```python
from build123d import *

# Parameters (mm, degrees)
F2_DEPTH = 38.1
F1_R     = 4.191664
F1_R_2   = 4.888278
F3_DEPTH = 38.1


with BuildPart() as f2:
    # F0 (on Front) → F2 (new body, symmetric)
    with BuildSketch(Plane.XZ):
        with BuildLine():
            Line((-53.521972, 29.483171), (-62.049322, 22.979138))
            Line((-62.049322, 22.979138), (-62.049322, -17.520668))
            Line((-62.049322, -17.520668), (-53.521972, -23.408599))
            Line((-53.521972, -23.408599), (-26.112633, -23.408599))
            Line((-26.112633, -23.408599), (-16.773155, -14.272154))
            Line((-16.773155, -14.272154), (1.499737, -21.175247))
            ThreePointArc((1.499737, -21.175247), (19.255094, -20.912232), (17.705545, -3.222666))
            Line((17.705545, -3.222666), (32.90997, 25.973593))
            ThreePointArc((32.90997, 25.973593), (50.002283, 33.973494), (41.596282, 50.869786))
            Line((41.596282, 50.869786), (15.718478, 59.210562))
            Line((15.718478, 59.210562), (-27.696349, 29.483171))
            Line((-27.696349, 29.483171), (-53.521972, 29.483171))
        make_face()
    extrude(amount=F2_DEPTH, both=True)

    # F1 (on face) → F3 (cut, symmetric)
    with BuildSketch(Plane.XZ):
        with Locations((10.020046, -12.490342)):
            Circle(F1_R)
        with Locations((38.078971, 39.35767)):
            Circle(F1_R_2)
        Polygon((-46.49493, -13.530695), (-34.363216, -6.82854), (-34.101594, 7.02891), (-45.971688, 14.184206), (-58.103403, 7.482052), (-58.365024, -6.375399), align=None)
    extrude(amount=F3_DEPTH, both=True, mode=Mode.SUBTRACT)


solid = f2.part
```
Here's how the part is built. I have some questions about the finished solid (model axes, mm). A direction names the side the tool comes from. Round coordinates to 2 decimals unless told otherwise and drop trailing zeros. Order: outer loops, then holes, each group sorted by start corner. A loop starts at its lowest first (then second) coordinate and runs counter-clockwise, first axis right, second up. Notation, with made-up numbers: M -8.75,79.5 L 49.25,79.5 A31 cw 49.25,104.5 Z; hole C 4.25,33.5 d4. An arc over 180 degrees is marked long. Use CSV: the item, a comma, the result in double quotes.
1) If we mould it in two halves opening along Z, with no side actions, what happens to faces 1 (the cylindrical face through (19.066, -0.533, -21.117)), 2 (the flat face through (-5.69, -0.53, 44.55)), 3 (the flat face through (-21.508, -0.533, -18.904)), 4 (the flat face through (25.2, -0.53, 11.17))? For each: pulls with the +Z half, pulls with the -Z half, needs draft (parallel to the pull), parting line crosses it, or undercut.
Taken from the geometry:
face 1,"undercut"
face 2,"pulls with the +Z half"
face 3,"pulls with the -Z half"
face 4,"undercut"
2) I want a section at B-B (x = 39.5). List the corners of the cut face in (y, z) for me.
Taken from the geometry:
outline,"M -38.1,25.27 L 38.1,25.27 L 38.1,34.68 L -38.1,34.68 Z; M -38.1,44.03 L 38.1,44.03 L 38.1,51.55 L -38.1,51.55 Z"
3) I want a section at C-C (y = 25). List the corners of the cut face in (x, z) for me, then the cut area to 3 significant figures.
Taken from the geometry:
outline,"M -62.05,-17.52 L -53.52,-23.41 L -26.11,-23.41 L -16.77,-14.27 L 1.5,-21.18 A12.12 ccw long 17.71,-3.22 L 32.91,25.97 A13.19 ccw long 41.6,50.87 L 15.72,59.21 L -27.7,29.48 L -53.52,29.48 L -62.05,22.98 Z; hole M -58.37,-6.38 L -46.49,-13.53 L -34.36,-6.83 L -34.1,7.03 L -45.97,14.18 L -58.1,7.48 Z; hole C 10.02,-12.49 d8.38; hole C 38.08,39.36 d9.78"
area,"5,250 mm^2"
4) I want a section at A-A (z = 37.5). List the corners of the cut face in (x, y) for me.
Taken from the geometry:
outline,"M -15.99,-38.1 L 33.56,-38.1 L 33.56,38.1 L -15.99,38.1 Z; M 42.6,-38.1 L 50.71,-38.1 L 50.71,38.1 L 42.6,38.1 Z"
5) On a 3-axis mill with a long thin cutter (end or side, diameter ignored), from which of +Z, -Z, +X, -X, +Y, -Y can I reach the whole of each face in a straight line? I mean faces 5 (the flat face through (-6, -38.1, 18)), 6 (the flat face through (-6, 38.1, 18)), 7 (the flat face through (-40, -1, -23.409)), 8 (the flat face through (-51.95, -0.53, 10.88)), 9 (the flat face through (-7.765, -0.533, -17.675)). Say none if no direction works.
Taken from the geometry:
face 5,"+Z, -Z, +X, -X, -Y"
face 6,"+Z, -Z, +X, -X, +Y"
face 7,"-Z, -X, +Y, -Y"
face 8,"+Y, -Y"
face 9,"-Z, +Y, -Y"
6) I'm going to push flat-ended pins straight in: P1, Ø5, axis at y = -14, z = 33.5, coming from the -X side; P2, Ø8, axis at x = -39, y = -18.5, coming from the -Z side; P3, Ø5, axis at x = 32, y = -21, coming from the +Z side; P4, Ø12.5, axis at x = 38.08, z = 39.36, coming from the -Y side. Where does each tip first touch, or does it pass through?
Taken from the geometry:
P1,"x = -25.48"
P2,"z = -23.41"
P3,"z = 54.77"
P4,"y = -38.1"
7) I need wall thicknesses on line 1 along X through (y, z) = (-29.5, -12); line 2 along X through (y, z) = (7.5, -10.5); line 3 along Z through (x, y) = (36, -15.5). Which ranges of each line are inside material? Lowest first, please. Write a range as [from, to].
Taken from the geometry:
line 1,"[-62.05, -49.03], [-43.72, 5.86], [14.18, 22.35]"
line 2,"[-62.05, -51.52], [-41.01, 6.33], [13.71, 22.16]"
line 3,"[25.22, 34.93], [43.78, 52.67]"
8) I want a section at D-D (z = 18.5). List the corners of the cut face in (x, y) for me, then the cut area to 3 significant figures.
Taken from the geometry:
outline,"M -62.05,-38.1 L 29.02,-38.1 L 29.02,38.1 L -62.05,38.1 Z"
area,"6,940 mm^2"
